from build123d import *

# Parameters (mm, degrees)
F0_W     = 95
F0_H     = 39.5
F1_DEPTH = 4.8
F2_R     = 8
F2_R_2   = 1.15
F3_DEPTH = 2.4
F4_R     = 9


with BuildPart() as f1:
    # F0 (on Top) → F1 (new body)
    with BuildSketch(Plane.XY):
        with Locations((35.675943, 8.646622)):
            Rectangle(F0_W, F0_H)
    extrude(amount=F1_DEPTH)

    # F2 (on face) → F3 (cut)
    with BuildSketch(Plane.XY.offset(4.8)):
        with Locations((0, 18)):
            Circle(F2_R)
        with Locations((0, 14)):
            Circle(F2_R_2, mode=Mode.SUBTRACT)
        with Locations((-4, 18)):
            Circle(F2_R_2, mode=Mode.SUBTRACT)
        with Locations((4, 18)):
            Circle(F2_R_2, mode=Mode.SUBTRACT)
        with Locations((18, 18)):
            Circle(F2_R)
        with Locations((18, 14)):
            Circle(F2_R_2, mode=Mode.SUBTRACT)
        with Locations((14, 18)):
            Circle(F2_R_2, mode=Mode.SUBTRACT)
        with Locations((22, 18)):
            Circle(F2_R_2, mode=Mode.SUBTRACT)
        with Locations((36, 18)):
            Circle(F2_R)
        with Locations((32, 18)):
            Circle(F2_R_2, mode=Mode.SUBTRACT)
        with Locations((36, 14)):
            Circle(F2_R_2, mode=Mode.SUBTRACT)
        with Locations((40, 18)):
            Circle(F2_R_2, mode=Mode.SUBTRACT)
        with Locations((54, 18)):
            Circle(F2_R)
        with Locations((54, 14)):
            Circle(F2_R_2, mode=Mode.SUBTRACT)
        with Locations((50, 18)):
            Circle(F2_R_2, mode=Mode.SUBTRACT)
        with Locations((58, 18)):
            Circle(F2_R_2, mode=Mode.SUBTRACT)
        with Locations((72, 18)):
            Circle(F2_R)
        with Locations((68, 18)):
            Circle(F2_R_2, mode=Mode.SUBTRACT)
        with Locations((72, 14)):
            Circle(F2_R_2, mode=Mode.SUBTRACT)
        with Locations((76, 18)):
            Circle(F2_R_2, mode=Mode.SUBTRACT)
        with Locations((72, 0)):
            Circle(F2_R)
        with Locations((72, -4)):
            Circle(F2_R_2, mode=Mode.SUBTRACT)
        with Locations((68, 0)):
            Circle(F2_R_2, mode=Mode.SUBTRACT)
        with Locations((76, 0)):
            Circle(F2_R_2, mode=Mode.SUBTRACT)
        with Locations((54, 0)):
            Circle(F2_R)
        with Locations((54, -4)):
            Circle(F2_R_2, mode=Mode.SUBTRACT)
        with Locations((50, 0)):
            Circle(F2_R_2, mode=Mode.SUBTRACT)
        with Locations((58, 0)):
            Circle(F2_R_2, mode=Mode.SUBTRACT)
        with Locations((36, 0)):
            Circle(F2_R)
        with Locations((32, 0)):
            Circle(F2_R_2, mode=Mode.SUBTRACT)
        with Locations((36, -4)):
            Circle(F2_R_2, mode=Mode.SUBTRACT)
        with Locations((40, 0)):
            Circle(F2_R_2, mode=Mode.SUBTRACT)
        with Locations((18, 0)):
            Circle(F2_R)
        with Locations((18, -4)):
            Circle(F2_R_2, mode=Mode.SUBTRACT)
        with Locations((14, 0)):
            Circle(F2_R_2, mode=Mode.SUBTRACT)
        with Locations((22, 0)):
            Circle(F2_R_2, mode=Mode.SUBTRACT)
        Circle(F2_R)
        with Locations((0, -4)):
            Circle(F2_R_2, mode=Mode.SUBTRACT)
        with Locations((-4, 0)):
            Circle(F2_R_2, mode=Mode.SUBTRACT)
        with Locations((4, 0)):
            Circle(F2_R_2, mode=Mode.SUBTRACT)
    extrude(amount=-F3_DEPTH, mode=Mode.SUBTRACT)

    # F4
    f4_edges = [f1.edges().sort_by_distance(p)[0] for p in [
        (-11.824057, -11.103378, 2.4),
        (-11.824057, 28.396622, 2.4),
        (83.175943, -11.103378, 2.4),
        (83.175943, 28.396622, 2.4),
    ]]
    fillet(f4_edges, radius=F4_R)


solid = f1.part
Source: CAD feature listing. Evaluate the final solid. Frame: model axes, mm. A direction names the side the tool comes from. Round coordinates to 2 decimals unless told otherwise and drop trailing zeros. Loops run counter-clockwise (first coordinate to the right, second up) from the corner with the lowest first, then second, coordinate; pieces in that order, holes last. Notation, with made-up numbers: (63, -17.5) - (120, -17.5) arc R5 ccw to (120, -12.5) - close; hole circle Ø6 at (51.5, 85). An arc over 180 degrees is marked (long way). Write item = value, one per line. Start each with the question number.
(1) Section query B-B, the plane x = 18. Output: boundary loops of the cut face in (y, z).
(2) Section query A-A, the plane z = 1.1. Output: boundary loops of the cut face in (x, y).
(3) Section query C-C, the plane y = 6.5. Output: boundary loops of the cut face in (x, z).
(4) Ray query, line 1 along Y through (x, z) = (36, 4.05); line 2 along X through (y, z) = (-6, 4.4); line 3 along X through (y, z) = (-7, 4.3). Return the intervals inside material, ascending. Write a range as from..to.
(5) Pin query (flat end, axial travel): pin 1 (5 mm diameter, centred on x = 18, y = 3.5, fed in from +Z). Return the tip coordinate at first contact, or that it passes through.
(6) Set-up query: faces 4 (the face through (-4, 0, 4.8)), 5 (the face through (2.85, 0.05, 3.62)). Return all of +Z, -Z, +X, -X, +Y, -Y with unobstructed straight access to the full face (end or side cutting, diameter ignored); none if empty.
(7) Pull-direction query (X, two-part tool) for faces 1 (the face through (18, 0, 2.4)), 2 (the face through (37.062, 13.56, 3.617)), 3 (the face through (4, 18, 4.8)); classes: +X half, -X half, draft (parallel to the pull), parting line (faces both ways), or undercut.
(8) Section query D-D, the plane x = 68. Output: boundary loops of the cut face in (y, z), plus the area to 3 significant figures.
Conclusion:
q1.outline = (-11.1, 0) - (28.4, 0) - (28.4, 4.8) - (26, 4.8) - (26, 2.4) - (15.15, 2.4) - (15.15, 4.8) - (12.85, 4.8) - (12.85, 2.4) - (10, 2.4) - (10, 4.8) - (8, 4.8) - (8, 2.4) - (-2.85, 2.4) - (-2.85, 4.8) - (-5.15, 4.8) - (-5.15, 2.4) - (-8, 2.4) - (-8, 4.8) - (-11.1, 4.8) - close
q2.outline = (-11.82, -2.1) arc R9 ccw to (-2.82, -11.1) - (74.18, -11.1) arc R9 ccw to (83.18, -2.1) - (83.18, 19.4) arc R9 ccw to (74.18, 28.4) - (-2.82, 28.4) arc R9 ccw to (-11.82, 19.4) - close
q3.outline = (-11.82, 0) - (83.18, 0) - (83.18, 4.8) - (76.66, 4.8) - (76.66, 2.4) - (67.34, 2.4) - (67.34, 4.8) - (58.66, 4.8) - (58.66, 2.4) - (49.34, 2.4) - (49.34, 4.8) - (40.66, 4.8) - (40.66, 2.4) - (31.34, 2.4) - (31.34, 4.8) - (22.66, 4.8) - (22.66, 2.4) - (13.34, 2.4) - (13.34, 4.8) - (4.66, 4.8) - (4.66, 2.4) - (-4.66, 2.4) - (-4.66, 4.8) - (-11.82, 4.8) - close
q4.line_1 = -11.1..-8, -5.15..-2.85, 8..10, 12.85..15.15, 26..28.4
q4.line_2 = -10.94..-5.29, 5.29..12.71, 23.29..30.71, 41.29..48.71, 59.29..66.71, 77.29..82.29
q4.line_3 = -10.38..-3.87, 3.87..14.13, 21.87..32.13, 39.87..50.13, 57.87..68.13, 75.87..81.73
q5.pin_1 = 2.4
q6.face_4 = +Z, +X, -X, +Y, -Y
q6.face_5 = +Z
q7.face_1 = undercut
q7.face_2 = undercut
q7.face_3 = draft
q8.outline = (-11.1, 0) - (28.4, 0) - (28.4, 4.8) - (24.93, 4.8) - (24.93, 2.4) - (19.15, 2.4) - (19.15, 4.8) - (16.85, 4.8) - (16.85, 2.4) - (11.07, 2.4) - (11.07, 4.8) - (6.93, 4.8) - (6.93, 2.4) - (1.15, 2.4) - (1.15, 4.8) - (-1.15, 4.8) - (-1.15, 2.4) - (-6.93, 2.4) - (-6.93, 4.8) - (-11.1, 4.8) - close
q8.area = 134 mm2
